```python
from build123d import *

# Parameters (mm, degrees)
SKETCH1_R           = 2.778125
BOSS_EXTRUDE1_DEPTH = 0.762


with BuildPart() as part:
    # Sketch1 → Boss-Extrude1 (new body)
    with BuildSketch(Plane(origin=(0, 0, 0), x_dir=(1, 0, 0), z_dir=(0, 1, 0))):
        with BuildLine():
            Line((-16.691428571, 19.145657791), (-32.475714286, 5.384716254))
            ThreePointArc((-32.475714286, 5.384716254), (-34.925, 0), (-32.475714286, -5.384716254))
            Line((-32.475714286, -5.384716254), (-16.691428571, -19.145657791))
            ThreePointArc((-16.691428571, -19.145657791), (0, -25.4), (16.691428571, -19.145657791))
            Line((16.691428571, -19.145657791), (32.475714286, -5.384716254))
            ThreePointArc((32.475714286, -5.384716254), (34.925, 0), (32.475714286, 5.384716254))
            Line((32.475714286, 5.384716254), (16.691428571, 19.145657791))
            ThreePointArc((16.691428571, 19.145657791), (0, 25.4), (-16.691428571, 19.145657791))
        make_face()
        with Locations(Location((-27.78125, 0, 0), (0, 0, 90))):
            Circle(SKETCH1_R, mode=Mode.SUBTRACT)
        with Locations(Location((27.78125, 0, 0), (0, 0, 90))):
            Circle(SKETCH1_R, mode=Mode.SUBTRACT)
    extrude(amount=BOSS_EXTRUDE1_DEPTH)

    # Sketch2 → Revolve1 (revolve)
    with BuildSketch(Plane.XY, mode=Mode.PRIVATE) as revolve1_sk:
        with BuildLine():
            Line((21.43125, 14.605), (21.43125, 0))
            Line((21.43125, 0), (0, 0))
            Line((0, 0), (0, 30.1625))
            ThreePointArc((0, 30.1625), (7.099515829, 27.992783709), (11.773215098, 22.225))
            ThreePointArc((11.773215098, 22.225), (17.924272694, 20.090631215), (21.43125, 14.605))
        make_face()
    revolve(revolve1_sk.sketch.rotate(Axis((0, 0, 0), (0, 1, 0)), 90), axis=Axis((0, 0, 0), (0, 1, 0)))


solid = part.part
```
The model under review builds one solid part; all positions refer to its coordinate system, in mm. A direction names the side the tool comes from. Round coordinates to 2 decimals unless told otherwise and drop trailing zeros. Loops run counter-clockwise (first coordinate to the right, second up) from the corner with the lowest first, then second, coordinate; pieces in that order, holes last. Notation, with made-up numbers: (-15.75, 32) - (-7.75, 32) arc R15 ccw to (-7.75, 59) - close; hole circle Ø6 at (67.25, 79.5). An arc over 180 degrees is marked (long way). Write each question's results on one line, items separated by ' | '. Start each with the question number.
Q1. Take a section at B-B on x = 0. Give the boundary of the cut face in (y, z) (1 decimal).
Q2. Take a section at D-D on y = 3. Give the boundary of the cut face in (x, z).
Q3. Tool access review of faces 1 (the cylindrical face through (-14.48, 7.59, 15.8)), 2 (the cylindrical face through (-0.3, 0.4, 25.4)): name each direction out of +Z, -Z, +X, -X, +Y, -Y from which nothing blocks a thin tool from reaching the whole face with its end or side.
Q4. Draft analysis for pull direction Z (two halves, no side actions). For faces 3 (the cylindrical face through (30.493, 0.376, 0.602)), 4 (the flat face through (-24.473, 0.376, -12.362)), 5 (the flat face through (0, 0, 0)), 6 (the cylindrical face through (34.924, 0.376, 0.085)), state which applies: pulls with the +Z half, pulls with the -Z half, needs draft (parallel to the pull), parting line crosses it, or undercut.
Q5. Take a section at C-C on y = 21. Give the boundary of the cut face in (x, z), plus the area to 3 significant figures.
Q6. Take a section at A-A on z = 0. Give the boundary of the cut face in (x, y) (1 decimal).
Q7. Wall thickness on line 1 along X through (y, z) = (0.55, 0) (3 decimals); line 2 along Y through (x, z) = (-27, 9); line 3 along Z through (x, y) = (5.5, 4): over which ranges is each line inside the solid? List them lowest first. Write a range as [from, to].
Q8. Insertion check: P1, Ø12, axis at x = -7, y = 9, coming from the +Z side; P2, Ø15, axis at x = 8, z = 6, coming from the +Y side; P3, Ø6, axis at x = 28, z = 5, coming from the -Y side; P4, Ø12, axis at x = 11, y = 19, coming from the +Z side. Each pin has a flat end and moves straight along its axis. Give the tip position at first contact, or say it passes through.
Data:
1) outline: (0, -25.4) - (0.8, -25.4) - (0.8, -21.4) - (14.6, -21.4) arc R9.9 ccw to (22.2, -11.8) arc R12.7 ccw to (22.2, 11.8) arc R9.9 ccw to (14.6, 21.4) - (0.8, 21.4) - (0.8, 25.4) - (0, 25.4) - close
2) outline: circle Ø42.86 at (0, 0)
3) face 1: +Y | face 2: +Z, +Y, -Y
4) face 3: undercut | face 4: pulls with the -Z half | face 5: needs draft | face 6: parting line crosses it
5) outline: circle Ø33.1 at (0, 0) | area: 861 mm²
6) outline: (-34.9, 0) - (-30.6, 0) - (-30.6, 0.8) - (-34.9, 0.8) - close; (-25, 0) - (25, 0) - (25, 0.8) - (21.4, 0.8) - (21.4, 14.6) arc R9.9 ccw to (11.8, 22.2) arc R12.7 ccw to (-11.8, 22.2) arc R9.9 ccw to (-21.4, 14.6) - (-21.4, 0.8) - (-25, 0.8) - close; (30.6, 0) - (34.9, 0) - (34.9, 0.8) - (30.6, 0.8) - close
7) line 1: x = [-34.925, -30.559], [-25.003, 25.003], [30.559, 34.925] | line 2: y = [0, 0.76] | line 3: z = [-20.71, 20.71]
8) P1: stops at z = 21.41 | P2: stops at y = 29.91 | P3: stops at y = 0 | P4: stops at z = 20.3
